Model file for the job. Use its own axes, mm. A direction names the side the tool comes from. Coordinates: 2 decimals unless noted, no trailing zeros. Write each loop counter-clockwise with the first axis right and the second up, starting at its lowest first coordinate (ties: lowest second). Pieces come first, ordered by that corner, then holes.
Q1. Drill centre lines: probe 1 along Y at (x, z) = (5, 1); probe 2 along Z at (x, y) = (9.5, -10); probe 3 along X at (y, z) = (8.5, 1.45). Where is each one in solid material? Low to high.
Q2. Band-saw the part on C-C, the plane x = -10. Write the cut outline in (y, z), plus the area to 3 significant figures.
Q3. Band-saw the part on A-A, the plane y = 0. Write the cut outline in (x, z), plus the area to 3 significant figures.
Q4. Band-saw the part on B-B, the plane x = 0. Write the cut outline in (y, z).
Q5. Pin check, flat tips, straight feed: P1, Ø0.8, axis at y = -9.5, z = 2, coming from the +X side; P2, Ø0.5, axis at y = -5, z = 2.5, coming from the +X side; P3, Ø5, axis at x = 13.5, y = -11, coming from the +Z side. Stop position of each tip, or through.
Q6. Band-saw the part on D-D, the plane z = 2.2. State how many separate pieces and enclosed holes the cut face has, plus the area to 3 significant figures.
Q7. Which spindle directions (+Z, -Z, +X, -X, +Y, -Y) get a long thin tool onto all of the face, cutting with end or side? Do faces 5 (the flat face through (-9.404, -4, 2)), 6 (the flat face through (-3, 1.581, 2)), 7 (the flat face through (-2, 0, -1)). Say none if no direction does.
Q8. Pull direction X, two halves, no side cores. Call faces 1 (the flat face through (-3, 6, 3)), 2 (the flat face through (9.806, 0, 2)), 3 (the flat face through (-3.747, -9.4, 2.2)), 4 (the cylindrical face through (-4.769, -21.477, 0.74)): released by +X, released by -X, zero draft, split by the parting line, or undercut.
from build123d import *

# Parameters (mm, degrees)
SKETCH_1_R          = 22
EXTRUDE_1_DEPTH     = 1.5
SKETCH_2_W          = 4
SKETCH_2_H          = 5
EXTRUDE_2_DEPTH     = 1.8
SKETCH_3_R          = 1
CUT_EXTRUDE_1_DEPTH = 1.8
SKETCH_4_W          = 7.015976939
SKETCH_4_H          = 6.325009514
SKETCH_4_W_2        = 4.916498991
SKETCH_4_H_2        = 11.400962527
SKETCH_4_W_3        = 1.886872586
SKETCH_4_H_3        = 0.903572787
SKETCH_4_W_4        = 0.637816086
SKETCH_4_H_4        = 1.036451139
SKETCH_4_W_5        = 0.744118766
SKETCH_4_W_6        = 0.797270107
SKETCH_4_W_7        = 0.690967426
SKETCH_4_H_5        = 1.833721246
EXTRUDE_3_DEPTH     = 1.5


with BuildPart() as part:
    # 草图1 → 凸台-拉伸1 (new body)
    with BuildSketch(Plane.XY):
        Circle(SKETCH_1_R)
    extrude(amount=EXTRUDE_1_DEPTH)

    # 草图2 → 凸台-拉伸2 (add)
    with BuildSketch(Plane(origin=(0, 0, 0), x_dir=(-1, 0, 0), z_dir=(0, 0, -1))):
        Rectangle(SKETCH_2_W, SKETCH_2_H)
    extrude(amount=EXTRUDE_2_DEPTH)

    # 草图3 → 切除-拉伸1 (cut)
    with BuildSketch(Plane(origin=(0, 0, 0), x_dir=(-1, 0, 0), z_dir=(0, 0, -1))):
        with Locations((10, 0)):
            Circle(SKETCH_3_R)
        with Locations((-5, 8.660254038)):
            Circle(SKETCH_3_R)
        with Locations((-5, -8.660254038)):
            Circle(SKETCH_3_R)
    extrude(amount=-CUT_EXTRUDE_1_DEPTH, mode=Mode.SUBTRACT)

    # 草图4 → 凸台-拉伸3 (add)
    with BuildSketch(Plane.XY.offset(1.5)):
        Polygon((-8.105579419, -3.654154656), (-6.654300112, -3.654154656), (-6.654300112, -4.661389837), (-7.070508219, -4.661389837), (-7.070508219, -5.140659778), (-7.379939766, -5.140659778), (-7.379939766, -4.661389837), (-7.726351297, -4.661389837), (-7.726351297, -5.140659778), (-7.991211002, -5.140659778), (-7.991211002, -4.661389837), (-8.331744908, -4.661389837), (-8.331744908, -5.140659778), (-8.747953015, -5.140659778), (-8.747953015, -4.661389837), (-9.403796093, -4.661389837), (-9.403796093, -3.654154656), align=None)
        with Locations((-3.003050736, 5.620754253)):
            Rectangle(SKETCH_4_W, SKETCH_4_H)
        with Locations((7.348172818, 0.345483713)):
            Rectangle(SKETCH_4_W_2, SKETCH_4_H_2)
        with Locations((-3.335246613, 1.129465985)):
            Rectangle(SKETCH_4_W_3, SKETCH_4_H_3)
        with Locations((-5.049377343, -9.38121159)):
            Rectangle(SKETCH_4_W_4, SKETCH_4_H_4)
        with Locations((-3.375110119, -9.38121159)):
            Rectangle(SKETCH_4_W_5, SKETCH_4_H_4)
        with Locations((-1.009875468, -9.38121159)):
            Rectangle(SKETCH_4_W_6, SKETCH_4_H_4)
        with Locations((3.747169502, -3.375110119)):
            Rectangle(SKETCH_4_W_7, SKETCH_4_H_5)
    extrude(amount=EXTRUDE_3_DEPTH)


solid = part.part
Answer sheet:
1. probe 1: y = -21.42 to -9.66, -7.66 to 7.66, 9.66 to 21.42
1. probe 2: z = 0 to 1.5
1. probe 3: x = -20.29 to 4.01, 5.99 to 20.29
2. outline: (-19.6, 0) - (-1, 0) - (-1, 1.5) - (-19.6, 1.5) - close; (1, 0) - (19.6, 0) - (19.6, 1.5) - (1, 1.5) - close
2. area: 55.8 mm2
3. outline: (-22, 0) - (-11, 0) - (-11, 1.5) - (-22, 1.5) - close; (-9, 0) - (-2, 0) - (-2, -1.8) - (2, -1.8) - (2, 0) - (22, 0) - (22, 1.5) - (9.81, 1.5) - (9.81, 3) - (4.89, 3) - (4.89, 1.5) - (-9, 1.5) - close
3. area: 77.6 mm2
4. outline: (-22, 0) - (-2.5, 0) - (-2.5, -1.8) - (2.5, -1.8) - (2.5, 0) - (22, 0) - (22, 1.5) - (8.78, 1.5) - (8.78, 3) - (2.46, 3) - (2.46, 1.5) - (-22, 1.5) - close
5. P1: stops at x = -0.61
5. P2: stops at x = 9.81
5. P3: stops at z = 1.5
6. separate pieces: 8
6. enclosed holes: 0
6. area: 109 mm2
7. face 5: +Z, -X, +Y, -Y
7. face 6: +Z, -X
7. face 7: -Z, -X, +Y, -Y
8. face 1: zero draft
8. face 2: released by +X
8. face 3: undercut
8. face 4: split by the parting line
